Could you check a few things on this model? Use its own coordinates, in mm. A direction names the side the tool comes from. Give positions to 0.01 mm unless a question says otherwise; leave off trailing zeros. Order: outer loops, then holes, each group sorted by start corner. A loop starts at its lowest first (then second) coordinate and runs counter-clockwise, first axis right, second up.
(1) Imagine slicing it at A-A, the plane x = 0. Write out the boundary of the cut face in (y, z), then the cut area to 3 significant figures.
(2) Imagine slicing it at C-C, the plane y = 10. Write out the boundary of the cut face in (x, z), then the cut area to 3 significant figures.
(3) If I drill on probe 1 along X at (y, z) = (1.95, 0); probe 2 along Y at (x, z) = (0, -9.1), over which ranges is the centre line in solid material (lowest first)?
(4) Imagine slicing it at D-D, the plane x = -6. Write out the boundary of the cut face in (y, z).
(5) If we mould it in two halves opening along Z, with no side actions, what happens to faces 1 (the cylindrical face through (-0.596, 1.619, 2.685)), 2 (the flat face through (-2.4, 7.6, -10)), 3 (the flat face through (-10, 3, -4))? For each: released by +Z, released by -Z, zero draft, split by the parting line, or undercut.
(6) Will these pins go through, and if not, where does the flat tip stop? pin 1 (10 mm diameter, centred on y = 7.5, z = 5, fed in from -X); pin 2 (1 mm diameter, centred on x = -6, z = 5, fed in from +Y); pin 3 (4.5 mm diameter, centred on x = 0.5, y = 9.5, fed in from +Z).
(7) Imagine slicing it at B-B, the plane z = 0. Write out the boundary of the cut face in (x, y), then the cut area to 3 significant figures.
(8) On a 3-axis mill with a long thin cutter (end or side, diameter ignored), from which of +Z, -Z, +X, -X, +Y, -Y can I reach the whole of each face in a straight line? I mean faces 4 (the flat face through (-2.4, 0, -2.4)), 5 (the flat face through (-2.4, 3.2, 2.1)). Say none if no direction works.
from build123d import *

# Parameters (mm, degrees)
SKETCH1_W           = 20
SKETCH1_H           = 20
BOSS_EXTRUDE1_DEPTH = 3.2
SKETCH2_W           = 20
SKETCH2_H           = 3.2
BOSS_EXTRUDE2_DEPTH = 16.8
SKETCH3_R           = 2.75
CUT_EXTRUDE1_DEPTH  = 4.2
SKETCH4_R           = 2.75
CUT_EXTRUDE2_DEPTH  = 4.2
FILLET1_R           = 2
FILLET2_R           = 0.25


with BuildPart() as part:
    # Sketch1 → Boss-Extrude1 (new body)
    with BuildSketch(Plane(origin=(0, 0, 0), x_dir=(1, 0, 0), z_dir=(0, 1, 0))):
        Rectangle(SKETCH1_W, SKETCH1_H)
    extrude(amount=BOSS_EXTRUDE1_DEPTH)

    # Sketch2 → Boss-Extrude2 (add)
    with BuildSketch(Plane(origin=(0, 3.2, 0), x_dir=(1, 0, 0), z_dir=(0, 1, 0))):
        with Locations((0, 8.4)):
            Rectangle(SKETCH2_W, SKETCH2_H)
    extrude(amount=BOSS_EXTRUDE2_DEPTH)

    # Sketch3 → Cut-Extrude1 (cut, through all)
    with BuildSketch(Plane(origin=(0, 3.2, 0), x_dir=(1, 0, 0), z_dir=(0, 1, 0))):
        Circle(SKETCH3_R)
    extrude(amount=-CUT_EXTRUDE1_DEPTH, mode=Mode.SUBTRACT)

    # Sketch4 → Cut-Extrude2 (cut, through all)
    with BuildSketch(Plane.XY.offset(-6.8)):
        with Locations((0, 10)):
            Circle(SKETCH4_R)
    extrude(amount=-CUT_EXTRUDE2_DEPTH, mode=Mode.SUBTRACT)

    # Fillet1
    fillet1_edges = [part.edges().sort_by_distance(p)[0] for p in [
        (0, 3.2, 10),
        (0, 20, -6.8),
    ]]
    fillet(fillet1_edges, radius=FILLET1_R)

    # Fillet2
    fillet2_edges = [part.edges().sort_by_distance(p)[0] for p in [
        (-2.75, 0, 0),
        (-2.75, 3.2, 0),
        (-2.75, 10, -10),
        (-2.75, 10, -6.8),
    ]]
    fillet(fillet2_edges, radius=FILLET2_R)


solid = part.part
Answer block:
1. outline: (0, -10) - (7, -10) arc R0.25 ccw to (7.25, -9.75) - (7.25, -7.05) arc R0.25 ccw to (7, -6.8) - (3.2, -6.8) - (3.2, -3) arc R0.25 ccw to (2.95, -2.75) - (0.25, -2.75) arc R0.25 ccw to (0, -3) - close; (0, 3) arc R0.25 ccw to (0.25, 2.75) - (2.95, 2.75) arc R0.25 ccw to (3.2, 3) - (3.2, 8) arc R2 ccw to (1.2, 10) - (0, 10) - close; (12.75, -9.75) arc R0.25 ccw to (13, -10) - (20, -10) - (20, -8.8) arc R2 ccw to (18, -6.8) - (13, -6.8) arc R0.25 ccw to (12.75, -7.05) - close
1. area: 80.7 mm2
2. outline: (-10, -10) - (-3, -10) arc R0.25 ccw to (-2.75, -9.75) - (-2.75, -7.05) arc R0.25 ccw to (-3, -6.8) - (-10, -6.8) - close; (2.75, -9.75) arc R0.25 ccw to (3, -10) - (10, -10) - (10, -6.8) - (3, -6.8) arc R0.25 ccw to (2.75, -7.05) - close
2. area: 46.3 mm2
3. probe 1: x = -10 to -2.75, 2.75 to 10
3. probe 2: y = 0 to 7.25, 12.75 to 20
4. outline: (0, -10) - (20, -10) - (20, -8.8) arc R2 ccw to (18, -6.8) - (3.2, -6.8) - (3.2, 8) arc R2 ccw to (1.2, 10) - (0, 10) - close
5. face 1: undercut
5. face 2: released by -Z
5. face 3: zero draft
6. pin 1: stops at x = -10
6. pin 2: stops at y = 3.2
6. pin 3: stops at z = -6.8
7. outline: (-10, 0) - (-3, 0) arc R0.25 ccw to (-2.75, 0.25) - (-2.75, 2.95) arc R0.25 ccw to (-3, 3.2) - (-10, 3.2) - close; (2.75, 0.25) arc R0.25 ccw to (3, 0) - (10, 0) - (10, 3.2) - (3, 3.2) arc R0.25 ccw to (2.75, 2.95) - close
7. area: 46.3 mm2
8. face 4: +Z, -Z, +X, -X, -Y
8. face 5: +Z, +X, -X, +Y
